```python
from build123d import *

# Parameters (mm, degrees)
SKETCH_1_W          = 33
SKETCH_1_H          = 30
EXTRUDE_1_DEPTH     = 4
SHELL_1_T           = -0.5
CUT_EXTRUDE_2_DEPTH = 1


with BuildPart() as part:
    # 草图1 → 拉伸1 (new body)
    with BuildSketch(Plane(origin=(0, 0, 0), x_dir=(1, 0, 0), z_dir=(0, 1, 0))):
        Rectangle(SKETCH_1_W, SKETCH_1_H)
    extrude(amount=EXTRUDE_1_DEPTH)

    # 抽壳1
    shell_1_openings = [part.faces().sort_by_distance(p)[0] for p in [
        (0, 2, -15),
    ]]
    offset(amount=SHELL_1_T, openings=shell_1_openings, kind=Kind.INTERSECTION)

    # 草图2 → 切除-拉伸2 (cut)
    with BuildSketch(Plane(origin=(0, 4, 0), x_dir=(-1, 0, 0), z_dir=(0, 1, 0))):
        with BuildLine():
            Line((10.985566132, -13.819893674), (10.985566132, 3.658083867))
            ThreePointArc((10.985566132, 3.658083867), (0, 5.904035161), (-10.985566132, 3.658083867))
            Line((-10.985566132, 3.658083867), (-10.985566132, -13.819893674))
            ThreePointArc((-10.985566132, -13.819893674), (0, -9.472380487), (10.985566132, -13.819893674))
        make_face()
    extrude(amount=-CUT_EXTRUDE_2_DEPTH, mode=Mode.SUBTRACT)


solid = part.part
```
Source: CAD feature listing. Evaluate the final solid. Frame: model axes, mm. A direction names the side the tool comes from. Give positions to 0.01 mm unless a question says otherwise; leave off trailing zeros. Loops run counter-clockwise (first coordinate to the right, second up) from the corner with the lowest first, then second, coordinate; pieces in that order, holes last. Notation, with made-up numbers: (47, -17.5) -> (68, -17.5) arc R23 ccw to (68, 7.5) -> close; hole circle Ø5 at (20.25, -15). An arc over 180 degrees is marked (long way). Use a Markdown table: item, result. Add a question column.
(1) Access query for faces 5 (the face through (-0.1, 3.8, -15)), 6 (the face through (0.169, 3.754, -9.473)), 7 (the face through (-16, 2, 0)). Directions: +Z, -Z, +X, -X, +Y, -Y. A direction counts if a zero-diameter tool reaches every point of the face in a straight line with its end or side. Return the directions, or none.
(2) Section query B-B (z = 12.25). Output: boundary loops of the cut face in (x, y), then the cut area to 3 significant figures.
(3) Ray query, line 1 (X direction, y = 1.3, z = -5); line 2 (Y direction, x = 9, z = 13.5); line 3 (Y direction, x = 6.5, z = -7.25). Return the intervals inside material, ascending.
(4) Section query A-A (x = 0). Output: boundary loops of the cut face in (y, z), then the cut area to 3 significant figures.
(5) First-contact query: pin 1 Ø1.5 at (x, y) = (0, 2.5) entering from -Z; pin 2 Ø2 at (x, z) = (0.5, 0.5) entering from +Y. Flat tips, straight axial feed; report the tip coordinate or a pass-through.
(6) Pull-direction query (X, two-part tool) for faces 1 (the face through (0, 0, 0)), 2 (the face through (0, 2, 14.5)), 3 (the face through (-0.158, 3.754, 5.904)), 4 (the face through (-16.5, 2, 0)); classes: +X half, -X half, draft (parallel to the pull), parting line (faces both ways), or undercut.
(7) Section query D-D (y = 2.3). Output: boundary loops of the cut face in (x, z), then the cut area to 3 significant figures.
(8) Section query C-C (x = -12). Output: boundary loops of the cut face in (y, z).
Checked values:
| question | item | result |
|---|---|---|
| 1 | face 5 | -Z, +X, -X, +Y, -Y |
| 1 | face 6 | +Y |
| 1 | face 7 | -Z |
| 2 | outline | (-16.5, 0) -> (16.5, 0) -> (16.5, 4) -> (-16.5, 4) -> close; hole (-16, 0.5) -> (16, 0.5) -> (16, 3.5) -> (-16, 3.5) -> close |
| 2 | area | 36.0 mm^2 |
| 3 | line 1 | -16.5 to -16, 16 to 16.5 |
| 3 | line 2 | 0 to 0.5, 3.5 to 4 |
| 3 | line 3 | 0 to 0.5 |
| 4 | outline | (0, -15) -> (0.5, -15) -> (0.5, 14.5) -> (3.5, 14.5) -> (3.5, 5.9) -> (4, 5.9) -> (4, 15) -> (0, 15) -> close; (3.5, -15) -> (4, -15) -> (4, -9.47) -> (3.5, -9.47) -> close |
| 4 | area | 23.8 mm^2 |
| 5 | pin 1 | z = 14.5 |
| 5 | pin 2 | y = 0.5 |
| 6 | face 1 | draft |
| 6 | face 2 | undercut |
| 6 | face 3 | undercut |
| 6 | face 4 | -X half |
| 7 | outline | (-16.5, -15) -> (-16, -15) -> (-16, 14.5) -> (16, 14.5) -> (16, -15) -> (16.5, -15) -> (16.5, 15) -> (-16.5, 15) -> close |
| 7 | area | 46.0 mm^2 |
| 8 | outline | (0, -15) -> (0.5, -15) -> (0.5, 14.5) -> (3.5, 14.5) -> (3.5, -15) -> (4, -15) -> (4, 15) -> (0, 15) -> close |
